from build123d import *

# Parameters (mm, degrees)
SKETCH1_R                                     = 8.89
TRAINGULAR_BASE_SIMPLIFIED_TO_CIRCLE_HE_DEPTH = 4
SKETCH2_R                                     = 5
DRIVE_SHAFT_DEPTH                             = 27.5
SKETCH4_R                                     = 5
SKETCH4_R_2                                   = 4.238
RETAINING_RING_SLOT_DEPTH                     = 1.143
HEX_SLOT_DEPTH                                = 11.049


with BuildPart() as part:
    # Sketch1 → Traingular base (simplified to circle here) (new body)
    with BuildSketch(Plane(origin=(0, 0, 0), x_dir=(1, 0, 0), z_dir=(0, 1, 0))):
        Circle(SKETCH1_R)
    extrude(amount=TRAINGULAR_BASE_SIMPLIFIED_TO_CIRCLE_HE_DEPTH)

    # Sketch2 → Drive shaft (add)
    with BuildSketch(Plane(origin=(0, 4, 0), x_dir=(1, 0, 0), z_dir=(0, 1, 0))):
        Circle(SKETCH2_R)
    extrude(amount=DRIVE_SHAFT_DEPTH)

    # Sketch4 → Retaining ring slot (cut)
    with BuildSketch(Plane(origin=(0, 16.7, 0), x_dir=(1, 0, 0), z_dir=(0, 1, 0))):
        Circle(SKETCH4_R)
        Circle(SKETCH4_R_2, mode=Mode.SUBTRACT)
    extrude(amount=RETAINING_RING_SLOT_DEPTH, mode=Mode.SUBTRACT)

    # Sketch5 → Hex slot (cut)
    with BuildSketch(Plane(origin=(0, 31.5, 0), x_dir=(1, 0, 0), z_dir=(0, 1, 0))):
        Polygon((3.6449, 0), (1.82245, 3.156575994), (-1.82245, 3.156575994), (-3.6449, 0), (-1.82245, -3.156575994), (1.82245, -3.156575994), align=None)
    extrude(amount=-HEX_SLOT_DEPTH, mode=Mode.SUBTRACT)


solid = part.part
Can you work these out from the model? Positions are in its coordinate system, mm. A direction names the side the tool comes from. Give positions to 0.01 mm unless a question says otherwise; leave off trailing zeros. Order: outer loops, then holes, each group sorted by start corner. A loop starts at its lowest first (then second) coordinate and runs counter-clockwise, first axis right, second up. Notation, with made-up numbers: M 61,84.25 L 66,84.25 A15 cw 66,90.25 Z; hole C 3.25,49.5 d11. An arc over 180 degrees is marked long. Use one line per item in the form item = value.
Item 1: If I drill on line 1 along Y through (x, z) = (-4, -6.75); line 2 along Z through (x, y) = (-3.25, 24); line 3 along Y through (x, z) = (2.25, -2), over which ranges is the centre line in solid material (lowest first)? Write a range as [from, to].
Values follow:
line_1 = [0, 4]
line_2 = [-3.8, -0.68], [0.68, 3.8]
line_3 = [0, 20.45]
Item 2: If we section it at B-B, the plane x = 0: Write out the boundary of the cut face in (y, z), and give its area (3 significant figures).
Values follow:
outline = M 0,-8.89 L 4,-8.89 L 4,-5 L 16.7,-5 L 16.7,-4.24 L 17.84,-4.24 L 17.84,-5 L 31.5,-5 L 31.5,-3.16 L 20.45,-3.16 L 20.45,3.16 L 31.5,3.16 L 31.5,5 L 17.84,5 L 17.84,4.24 L 16.7,4.24 L 16.7,5 L 4,5 L 4,8.89 L 0,8.89 Z
area = 275 mm^2
Item 3: If we section it at A-A, the plane y = 21: Write out the boundary of the cut face in (x, z), and give its area (3 significant figures).
Values follow:
outline = C 0,0 d10; hole M -3.64,0 L -1.82,-3.16 L 1.82,-3.16 L 3.64,0 L 1.82,3.16 L -1.82,3.16 Z
area = 44.0 mm^2
Item 4: If we section it at D-D, the plane y = 6: Write out the boundary of the cut face in (x, z), and give its area (3 significant figures).
Values follow:
outline = C 0,0 d10
area = 78.5 mm^2
Item 5: If we section it at C-C, the plane z = -0.5: Write out the boundary of the cut face in (x, y).
Values follow:
outline = M -8.88,0 L 8.88,0 L 8.88,4 L 4.97,4 L 4.97,16.7 L 4.21,16.7 L 4.21,17.84 L 4.97,17.84 L 4.97,31.5 L 3.36,31.5 L 3.36,20.45 L -3.36,20.45 L -3.36,31.5 L -4.97,31.5 L -4.97,17.84 L -4.21,17.84 L -4.21,16.7 L -4.97,16.7 L -4.97,4 L -8.88,4 Z
Item 6: Will these pins go through, and if not, where does the flat tip stop? pin 1 Ø1.5 at (x, y) = (-0.5, 21) entering from -Z; pin 2 Ø4 at (y, z) = (18, -1.5) entering from -X; pin 3 Ø1 at (x, z) = (0, 1.5) entering from +Y.
Values follow:
pin_1 = -5
pin_2 = -5
pin_3 = 20.45
Item 7: Thinking about a two-plate mould opening in X: for faces 1 (the flat face through (0, 20.451, 0)), 2 (the cylindrical face through (-1.08, 24.58, 4.88)), 3 (the flat face through (3.3, 31.5, 1)), which applies, pulls with the +X half, pulls with the -X half, needs draft (parallel to the pull), parting line crosses it, or undercut?
Values follow:
face_1 = undercut
face_2 = parting line crosses it
face_3 = needs draft
Item 8: For faces 4 (the flat face through (-4, 16.7, -2)), 5 (the flat face through (0, 0, 0)), 6 (the flat face through (0, 26, -3.157)), which set-ups out of +Z, -Z, +X, -X, +Y, -Y let a thin tool reach every point of the face, with its end or its side?
Values follow:
face_4 = none
face_5 = +Z, -Z, +X, -X, -Y
face_6 = +Y
